The model under review builds one solid part; all positions refer to its coordinate system, in mm. Face numbers are marked on the shaded views. A direction names the side the tool comes from. Give positions to 0.01 mm unless a question says otherwise; leave off trailing zeros. Order: outer loops, then holes, each group sorted by start corner. A loop starts at its lowest first (then second) coordinate and runs counter-clockwise, first axis right, second up. Notation, with made-up numbers: (25.25, -17.5) - (65.25, -17.5) arc R28 cw to (65.25, 0.5) - close; hole circle Ø8 at (77, -12). An arc over 180 degrees is marked (long way). Write item = value, one per line. Start each with the question number.
1. Machinability: for the marked faces 4 and 5, which of the approach directions +Z, -Z, +X, -X, +Y, -Y give a long, thin tool a straight path to every point of the face, cutting with its end or side? Answer none if there is none.
2. Mouldability with a two-part tool opening along Y and no side actions: class the marked faces 1, 2 and 3 as pulls with the +Y half, pulls with the -Y half, needs draft (parallel to the pull), parting line crosses it, or undercut.
3. We need section D-D, the plane x = -10. Give the boundary of the cut face in (y, z), and give its area (3 significant figures).
4. We need section C-C, the plane y = 12.7. Give the boundary of the cut face in (x, z) (3 decimals), and give its area (3 significant figures).
5. Wall thickness on probe 1 along Y at (x, z) = (6.5, 7.5); probe 2 along Z at (x, y) = (0, 22.75) (3 decimals); probe 3 along Z at (x, y) = (-12.5, 14.25): over which ranges is each line inside the solid? List them lowest first.
6. We need section A-A, the plane x = 0. Give the boundary of the cut face in (y, z) (3 decimals).
7. We need section B-B, the plane z = 7.5. Give the boundary of the cut face in (x, y).
8. For P1, Ø4, axis at x = -6.5, z = -7, coming from the -Y side; P2, Ø6, axis at y = 14.5, z = -37, coming from the +X side; P3, Ø5.5, axis at x = 0, z = 12.7, coming from the -Y side (3 decimals); P4, Ø8, axis at y = 3, z = -40, coming from the +X side, all flat-tipped, find the tip position at first contact; note any pin that passes through.
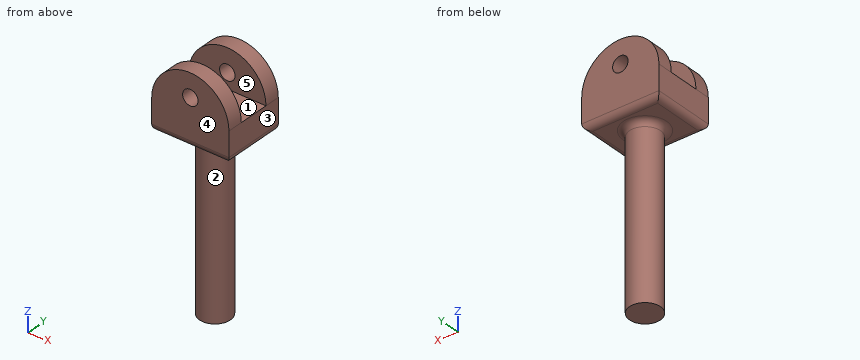
from build123d import *

# Parameters (mm, degrees)
F6_R     = 3.175
F0_DEPTH = 6.35
F6_W     = 31.75
F6_H     = 12.7
F1_DEPTH = 12.7
F3_R     = 6.35
F4_DEPTH = 76.2
F5_R     = 2.54


with BuildPart() as f0:
    # F6 (on Front) → F0 (new body)
    with BuildSketch(Plane.XZ):
        with BuildLine():
            Line((-15.875, 6.35), (15.875, 6.35))
            ThreePointArc((15.875, 6.35), (0, 22.225), (-15.875, 6.35))
        make_face()
        with Locations((0, 12.7)):
            Circle(F6_R, mode=Mode.SUBTRACT)
    extrude(amount=-F0_DEPTH)

    # F6 (on Front) → F1 (join)
    with BuildSketch(Plane.XZ):
        Rectangle(F6_W, F6_H)
    extrude(amount=-F1_DEPTH)

    # F2: F0 across face


with BuildPart() as f0_1:
    add(f0.part)
    add(f0.part.mirror(Plane(origin=(0, 12.7, 0), x_dir=(1, 0, 0), z_dir=(0, 1, 0))))

    # F3 (on Top) → F4 (join)
    with BuildSketch(Plane.XY):
        with Locations((0, 12.7)):
            Circle(F3_R)
    extrude(amount=-F4_DEPTH)

    # F5
    f5_edges = [f0_1.edges().sort_by_distance(p)[0] for p in [
        (-15.875, 12.7, -6.35),
        (0, 25.4, -6.35),
        (0, 0, -6.35),
        (15.875, 12.7, -6.35),
        (-6.35, 12.7, -6.35),
    ]]
    fillet(f5_edges, radius=F5_R)


solid = f0_1.part
Model answer:
q1.face_4 = +Z, -Z, +X, -X, -Y
q1.face_5 = +Z, +X, -X
q2.face_1 = undercut
q2.face_2 = parting line crosses it
q2.face_3 = needs draft
q3.outline = (0, -3.81) arc R2.54 ccw to (2.54, -6.35) - (22.86, -6.35) arc R2.54 ccw to (25.4, -3.81) - (25.4, 18.68) - (19.05, 18.68) - (19.05, 6.35) - (6.35, 6.35) - (6.35, 18.68) - (0, 18.68) - close
q3.area = 476 mm2
q4.outline = (-15.875, -3.81) arc R2.54 ccw to (-13.335, -6.35) - (-8.89, -6.35) arc R2.54 cw to (-6.35, -8.89) - (-6.35, -76.2) - (6.35, -76.2) - (6.35, -8.89) arc R2.54 cw to (8.89, -6.35) - (13.335, -6.35) arc R2.54 ccw to (15.875, -3.81) - (15.875, 6.35) - (-15.875, 6.35) - close
q4.area = 1,290 mm2
q5.probe_1 = 0 to 6.35, 19.05 to 25.4
q5.probe_2 = -6.35 to 9.525, 15.875 to 22.225
q5.probe_3 = -6.35 to 6.35
q6.outline = (0, -3.81) arc R2.54 ccw to (2.54, -6.35) - (3.81, -6.35) arc R2.54 cw to (6.35, -8.89) - (6.35, -76.2) - (19.05, -76.2) - (19.05, -8.89) arc R2.54 cw to (21.59, -6.35) - (22.86, -6.35) arc R2.54 ccw to (25.4, -3.81) - (25.4, 9.525) - (19.05, 9.525) - (19.05, 6.35) - (6.35, 6.35) - (6.35, 9.525) - (0, 9.525) - close; (0, 15.875) - (6.35, 15.875) - (6.35, 22.225) - (0, 22.225) - close; (19.05, 15.875) - (25.4, 15.875) - (25.4, 22.225) - (19.05, 22.225) - close
q7.outline = (-15.83, 0) - (15.83, 0) - (15.83, 6.35) - (-15.83, 6.35) - close; (-15.83, 19.05) - (15.83, 19.05) - (15.83, 25.4) - (-15.83, 25.4) - close
q8.P1 = 0.3
q8.P2 = 6.35
q8.P3 = through
q8.P4 = 2.8
